For this review, take the finished solid that the model builds, in its own axes (mm). A direction names the side the tool comes from. Round coordinates to 2 decimals unless told otherwise and drop trailing zeros. Write each loop counter-clockwise with the first axis right and the second up, starting at its lowest first coordinate (ties: lowest second). Pieces come first, ordered by that corner, then holes. Notation, with made-up numbers: (0.5, 52.25) - (9.5, 52.25) arc R30 ccw to (9.5, 91.25) - close; hole circle Ø3 at (-29.5, -28.5). An arc over 180 degrees is marked (long way). Answer in a Markdown table with one row per item. Add a question column.
from build123d import *

# Parameters (mm, degrees)
F0_R     = 4.7498
F0_R_2   = 2.460625
F0_R_3   = 12.1158
F0_R_4   = 11.049
F1_DEPTH = 8.8138
F2_R     = 7.62


with BuildPart() as f1:
    # F0 (on Top) → F1 (new body)
    with BuildSketch(Plane.XY):
        with BuildLine():
            ThreePointArc((22.424904, -33.259839), (42.551194, -11.399454), (48.252126, 17.762907))
            ThreePointArc((48.252126, 17.762907), (39.493301, 26.578964), (27.069985, 26.89691))
            Line((27.069985, 26.89691), (-8.001, 13.858139))
            ThreePointArc((-8.001, 13.858139), (-10.104465, 14.389846), (-10.355861, 16.544859))
            ThreePointArc((-10.355861, 16.544859), (1.261852, 29.673183), (17.591413, 36.050455))
            ThreePointArc((17.591413, 36.050455), (-11.40338, 42.550142), (-39.509192, 32.906113))
            ThreePointArc((-39.509192, 32.906113), (-42.764709, 20.91272), (-36.8284, 9.99484))
            Line((-36.8284, 9.99484), (-8.001, -13.858139))
            ThreePointArc((-8.001, -13.858139), (-7.40974, -15.945647), (-9.150338, -17.240868))
            ThreePointArc((-9.150338, -17.240868), (-26.328657, -13.743796), (-40.016317, -2.790617))
            ThreePointArc((-40.016317, -2.790617), (-31.147814, -31.150688), (-8.742934, -50.669021))
            ThreePointArc((-8.742934, -50.669021), (3.271408, -47.491684), (9.758415, -36.891749))
            Line((9.758415, -36.891749), (16.002, 0))
            ThreePointArc((16.002, 0), (17.514205, 1.5558), (19.506198, 0.696009))
            ThreePointArc((19.506198, 0.696009), (25.066804, -15.929388), (22.424904, -33.259839))
        make_face()
        with Locations((-24.393054, -25.120101)):
            Circle(F0_R, mode=Mode.SUBTRACT)
        with Locations((-31.344392, -15.606719)):
            Circle(F0_R_2, mode=Mode.SUBTRACT)
        with Locations((-4.651044, -34.704587)):
            Circle(F0_R_3, mode=Mode.SUBTRACT)
        with Locations((0.333594, -17.319588)):
            Circle(F0_R, mode=Mode.SUBTRACT)
        Circle(F0_R_4, mode=Mode.SUBTRACT)
        with Locations((-27.729533, 21.380216)):
            Circle(F0_R_3, mode=Mode.SUBTRACT)
        with Locations((-15.166, 8.370893)):
            Circle(F0_R, mode=Mode.SUBTRACT)
        with Locations((-9.558119, 33.685055)):
            Circle(F0_R, mode=Mode.SUBTRACT)
        with Locations((2.156381, 34.948399)):
            Circle(F0_R_2, mode=Mode.SUBTRACT)
        with Locations((29.188011, -19.34168)):
            Circle(F0_R_2, mode=Mode.SUBTRACT)
        with Locations((33.951173, -8.564954)):
            Circle(F0_R, mode=Mode.SUBTRACT)
        with Locations((14.832406, 8.948695)):
            Circle(F0_R, mode=Mode.SUBTRACT)
        with Locations((32.380576, 13.324372)):
            Circle(F0_R_3, mode=Mode.SUBTRACT)
    extrude(amount=F1_DEPTH)

    # F2
    f2_edges = [f1.edges().sort_by_distance(p)[0] for p in [
        (-39.509192, 32.906113, 4.4069),
        (48.252126, 17.762907, 4.4069),
        (-8.742934, -50.669021, 4.4069),
    ]]
    fillet(f2_edges, radius=F2_R)


solid = f1.part
Q1. Draft analysis for pull direction X (two halves, no side actions). For faces 3 (the face through (-10.198, 42.603, 4.345)), 4 (the face through (-16.538, 16.74, 4.345)), state which applies: released by +X, released by -X, zero draft, split by the parting line, or undercut.
Q2. Add section B-B on x = 36. State the section outline as (y, z) points.
Q3. Add section D-D on z = 5.25. Count the separate pieces of the cut face and the enclosed holes in it, then the cut area to 3 significant figures.
Q4. Tool access review of faces 1 (the face through (-26.1, -13.85, 4.35)), 2 (the face through (38.715, 26.892, 4.345)): name each direction out of +Z, -Z, +X, -X, +Y, -Y from which nothing blocks a thin tool from reaching the whole face with its end or side.
Q5. Add section A-A on x = -2. State the section outline as (y, z) points.
Q6. To check wall thickness, follow probe 1 along Y at (x, z) = (2.5, 7); probe 2 along X at (y, z) = (-27, 6.5) (1 decimal); probe 3 along Y at (x, z) = (0, 2.75). State the ranges of each line that lie inside material, in increasing order.
Q7. Add section C-C on y = -32. State the section outline as (x, z) points, then the cut area to 3 significant figures.
Q8. Insertion check: pin 1 Ø2 at (x, z) = (19, 5) entering from +Y; pin 2 Ø4 at (x, z) = (-8.5, 5.5) entering from +Y; pin 3 Ø3 at (y, z) = (-12, 7.5) entering from +X. Each pin has a flat end and moves straight along its axis. Give the tip position at first contact, or say it passes through.
Answer sheet:
| question | item | result |
|---|---|---|
| 1 | face 3 | split by the parting line |
| 1 | face 4 | undercut |
| 2 | outline | (-21.43, 0) - (-12.85, 0) - (-12.85, 8.81) - (-21.43, 8.81) - close; (-4.28, 0) - (1.76, 0) - (1.76, 8.81) - (-4.28, 8.81) - close; (24.89, 0) - (27.65, 0) - (27.65, 8.81) - (24.89, 8.81) - close |
| 3 | separate pieces | 1 |
| 3 | enclosed holes | 13 |
| 3 | area | 2,750 mm² |
| 4 | face 1 | +Z, -Z |
| 4 | face 2 | +Z, -Z, +Y |
| 5 | outline | (-50.12, 0) - (-46.53, 0) - (-46.53, 8.81) - (-50.12, 8.81) - close; (-22.88, 0) - (-21.46, 0) - (-21.46, 8.81) - (-22.88, 8.81) - close; (-13.18, 0) - (-10.87, 0) - (-10.87, 8.81) - (-13.18, 8.81) - close; (10.87, 0) - (16.09, 0) - (16.09, 8.81) - (10.87, 8.81) - close; (27.12, 0) - (42.26, 0) - (42.26, 8.81) - (27.12, 8.81) - close |
| 6 | probe 1 | y = -48.03 to -44.48, -24.92 to -21.55, -13.09 to -10.76, 10.76 to 17.76, 30.5 to 32.51, 37.38 to 41.53 |
| 6 | probe 2 | x = -33.6 to -28.8, -20 to -14, 4.7 to 11.4, 24.4 to 30.7 |
| 6 | probe 3 | y = -49.39 to -45.89, -23.52 to -22.06, -12.58 to -11.05, 11.05 to 16.83, 28.75 to 33.76, 36.13 to 41.98 |
| 7 | outline | (-30.58, 0) - (-16.46, 0) - (-16.46, 8.81) - (-30.58, 8.81) - close; (7.16, 0) - (10.59, 0) - (10.59, 8.81) - (7.16, 8.81) - close; (22.91, 0) - (24.38, 0) - (24.38, 8.81) - (22.91, 8.81) - close |
| 7 | area | 168 mm² |
| 8 | pin 1 | stops at y = 24.27 |
| 8 | pin 2 | stops at y = 42.63 |
| 8 | pin 3 | stops at x = 43 |
